Autodesk Inventor part; units mm, degrees
ref_plane "Start Plane" through (0, 0, 0) normal (0, 0, 1) x (1, 0, 0)
ref_plane "End Plane" through (0, 0, 1000) normal (0, 0, 1) x (1, 0, 0)
ref_plane "Work Plane4" through (0, 12.7, 1000) normal (0.7071, 0, 0.7071) x (0.7071, 0, -0.7071)
ref_plane "Start Plane" through (0, 0, 0) normal (0, 0, 1) x (1, 0, 0)
ref_plane "End Plane" through (0, 0, 1000) normal (0, 0, 1) x (1, 0, 0)
sketch "Sketch" plane through (0, 0, 0) normal (0, 0, 1) x (1, 0, 0)
  line L0 (25.4, 0) -> (0, 0)
  line L1 (0, 0) -> (0, 25.4)
  line L2 (0, 25.4) -> (1.651, 25.4)
  line L3 (3.175, 23.876) -> (3.175, 6.477)
  line L4 (6.477, 3.175) -> (23.876, 3.175)
  line L5 (25.4, 1.651) -> (25.4, 0)
  line L6 (0, -11.0414) -> (0, 31.5385) construction
  line L7 (-11.0414, 0) -> (31.5385, 0) construction
  arc A0 (3.175, 6.477) -> (6.477, 3.175) centre (6.477, 6.477) ccw
  arc A1 (3.175, 23.876) -> (1.651, 25.4) centre (1.651, 23.876) ccw
  arc A2 (25.4, 1.651) -> (23.876, 3.175) centre (23.876, 1.651) ccw
  line L8 (0, 40.0545) -> (0, -19.5574) construction
  line L9 (-19.5574, 0) -> (40.0545, 0) construction
  point P0 (3.175, 25.4)
  point P1 (3.175, 3.175)
  point P2 (25.4, 3.175)
  dimension "d0" = 25.4
  dimension "d1" = 25.4
  dimension "d2" = 3.175
  dimension "d3" = 3.175
  dimension "d10" = 0
  dimension "d11" = 0
  dimension "d14" = 3.302
  dimension "d15" = 1.524
extrude "Body" add sketch "Sketch" along normal up to surface (1000 mm away) from surface at 0
sketch "Sketch3" plane through (0, 0, 0) normal (0, 0, 1) x (1, 0, 0)
  line L0 (0, 0) -> (10, 0)
ref_plane "Work Plane3" through (0, 0, 0) normal (0, -1, 0) x (1, 0, 0)
ref_plane "Work Plane4" through (0, 12.7, 1000) normal (0.7071, 0, 0.7071) x (0.7071, 0, -0.7071)
split "Split1" plane through (0, 12.7, 1000) removes the side toward (0.7071, 0, 0.7071)
ref_plane "Work Plane5" through (0, 12.7, 0) normal (0.7071, 0, -0.7071) x (-0.7071, 0, -0.7071)
split "Split2" plane through (0, 12.7, 0) removes the side toward (0.7071, 0, -0.7071)
sketch "Sketch4" plane through (0, 0, 0) normal (0, -1, 0) x (1, 0, 0)
  line L0 (-2, 0) -> (12, 0)
  line L1 (-2, 1000) -> (12, 1000)
  dimension "d17" = 1000
equation "\"d0\" = G_H"
equation "\"d1\" = G_H"
equation "\"d2\" = G_T"
equation "\"d3\" = G_T"
equation "\"d14\" = G_IR"
equation "\"d15\" = G_ER"
equation "\"d4\" = G_L"
equation "\"G_H\" = 25.4"
equation "\"G_T\" = 3.175"
equation "\"G_ER\" = 1.524"
equation "\"G_IR\" = 3.302"
equation "\"G_L\" = d17"
equation "\"ex\" = 0"
equation "\"G_OFFSET_START\" = 0"
equation "\"G_OFFSET_END\" = 0"
properties part number "AISC - L 1 x 1 x 1/8 - 39.37" material "Steel, Mild"
Design review of the part built by this model. Coordinates are the model's own, in mm. A direction names the side the tool comes from. Round coordinates to 2 decimals unless told otherwise and drop trailing zeros. Order: outer loops, then holes, each group sorted by start corner. A loop starts at its lowest first (then second) coordinate and runs counter-clockwise, first axis right, second up. Notation, with made-up numbers: M -28.5,-8 L 12.5,-8 A19 cw 12.5,14 Z; hole C 79.25,61.5 d8. An arc over 180 degrees is marked long. Answer as CSV lines item,"result". Start each with the question number.
1) For pin 1 Ø5 at (y, z) = (14.5, 363.5) entering from +X (3 decimals); pin 2 Ø1 at (x, z) = (4, 181.5) entering from +Y; pin 3 Ø5 at (x, z) = (16.5, 451) entering from +Y (3 decimals), all flat-tipped, find the tip position at first contact; note any pin that passes through.
2) Wall thickness on line 1 along Y through (x, z) = (21.25, 865.5) (3 decimals); line 2 along Z through (x, y) = (1.5, 8.25): over which ranges is each line inside the solid? List them lowest first. Write a range as [from, to].
3) Add section A-A (z = 349). Give the boundary of the cut face in (x, y) (3 decimals).
4) Tool access review of faces 4 (the face through (8, 2, 992)), 5 (the face through (15, 3.175, 493)): name each direction out of +Z, -Z, +X, -X, +Y, -Y from which nothing blocks a thin tool from reaching the whole face with its end or side.
5) Add section B-B (y = 14.25). Give the boundary of the cut face in (x, z) (3 decimals), then the cut area to 3 significant figures.
6) Add section C-C (x = 15). Give the boundary of the cut face in (y, z) (3 decimals).
7) The part is to be moulded in two halves that separate along X. For faces 1 (the face through (8, 2, 8)), 2 (the face through (0, 13, 493)), 3 (the face through (13, 0, 493)), say which applies: +X half, -X half, draft (parallel to the pull), parting line (faces both ways), or undercut.
Resolved:
1,pin 1,"x = 3.175"
1,pin 2,"y = 5.05"
1,pin 3,"y = 3.175"
2,line 1,"[0, 3.175]"
2,line 2,"[1.5, 998.5]"
3,outline,"M 0,0 L 25.4,0 L 25.4,1.651 A1.524 ccw 23.876,3.175 L 6.477,3.175 A3.302 cw 3.175,6.477 L 3.175,23.876 A1.524 ccw 1.651,25.4 L 0,25.4 Z"
4,face 4,"+Z, +X, +Y, -Y"
4,face 5,"+Z, -Z, +X, +Y"
5,outline,"M 0,0 L 3.175,3.175 L 3.175,996.825 L 0,1000 Z"
5,area,"3,160 mm^2"
6,outline,"M 0,15 L 3.175,15 L 3.175,985 L 0,985 Z"
7,face 1,"+X half"
7,face 2,"-X half"
7,face 3,"draft"
